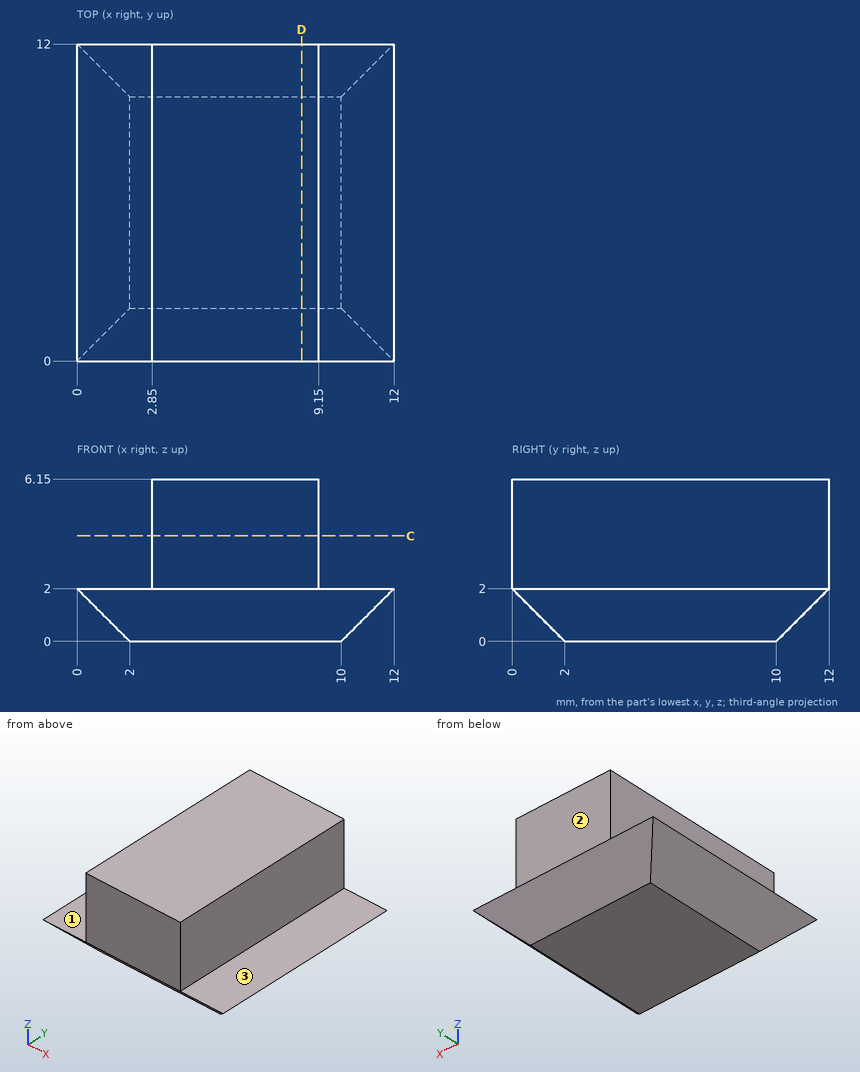
Answer from the drawing. Dimensions are ordinates in mm from the lowest x, y and z of the part. A direction names the side the tool comes from. Coordinates: 2 decimals unless noted, no trailing zeros. Loops run counter-clockwise (first coordinate to the right, second up) from the corner with the lowest first, then second, coordinate; pieces in that order, holes last.
Q1. Consider probe 1 along X at (y, z) = (5, 4.5); probe 2 along Y at (x, z) = (9.5, 0.75); probe 3 along Z at (x, y) = (1, 2.75). Determine where each line is inside the solid, lowest interval first.
Q2. The part is cut by section C-C on z = 4. Write down the section's boundary in (x, y).
Q3. Each of these flat-tipped pins is pushed along its axis until it touches: pin 1 Ø3.5 at (y, z) = (4.5, 3.5) entering from -X; pin 2 Ø3 at (x, y) = (1, 4) entering from +Z; pin 3 Ø2 at (y, z) = (5, 5) entering from +X. Where does it stop, or does it pass through?
Q4. The part is cut by section D-D on x = 8.5. Write down the section's boundary in (y, z).
Q5. Which of the six approach directions +Z, -Z, +X, -X, +Y, -Y give full straight-line access (tool end or side, diameter ignored) to the marked faces 1, 2 and 3?
Results below:
1. probe 1: x = 2.85 to 9.15
1. probe 2: y = 1.25 to 10.75
1. probe 3: z = 1 to 2
2. outline: (2.85, 0) - (9.15, 0) - (9.15, 12) - (2.85, 12) - close
3. pin 1: stops at x = 0
3. pin 2: stops at z = 2
3. pin 3: stops at x = 9.15
4. outline: (0, 2) - (2, 0) - (10, 0) - (12, 2) - (12, 6.15) - (0, 6.15) - close
5. face 1: +Z, -X, +Y, -Y
5. face 2: +Z, -Z, +X, -X, +Y
5. face 3: +Z, +X, +Y, -Y
